from build123d import *

# Parameters (mm, degrees)
F0_W     = 77.2
F0_H     = 152.5
F1_DEPTH = 10.9
F2_R     = 10
F3_R     = 8
F4_R     = 1


with BuildPart() as f1:
    # F0 (on Top) → F1 (new body)
    with BuildSketch(Plane.XY):
        Rectangle(F0_W, F0_H)
    extrude(amount=F1_DEPTH)

    # F2
    f2_edges = [f1.edges().sort_by_distance(p)[0] for p in [
        (38.6, 76.25, 5.45),
        (-38.6, 76.25, 5.45),
        (-38.6, -76.25, 5.45),
        (38.6, -76.25, 5.45),
    ]]
    fillet(f2_edges, radius=F2_R)

    # F3
    f3_edges = [f1.edges().sort_by_distance(p)[0] for p in [
        (0, -76.25, 10.9),
        (-35.671068, -73.321068, 10.9),
        (35.671068, -73.321068, 10.9),
        (-38.6, 0, 10.9),
        (38.6, 0, 10.9),
        (-35.671068, 73.321068, 10.9),
        (35.671068, 73.321068, 10.9),
        (0, 76.25, 10.9),
    ]]
    fillet(f3_edges, radius=F3_R)

    # F4
    f4_edges = [f1.edges().sort_by_distance(p)[0] for p in [
        (0, -76.25, 0),
        (-35.671068, -73.321068, 0),
        (35.671068, -73.321068, 0),
        (-38.6, 0, 0),
        (38.6, 0, 0),
        (-35.671068, 73.321068, 0),
        (35.671068, 73.321068, 0),
        (0, 76.25, 0),
    ]]
    fillet(f4_edges, radius=F4_R)


solid = f1.part
Geometry: final body of the model. Coordinates: model frame, mm. Coordinates: 2 decimals unless noted, no trailing zeros. Loops run counter-clockwise (first coordinate to the right, second up) from the corner with the lowest first, then second, coordinate; pieces in that order, holes last. Notation, with made-up numbers: (13, 80.5) - (28, 80.5) arc R8 cw to (28, 89.5) - close; hole circle Ø11 at (-18, -18.5). An arc over 180 degrees is marked (long way). Put each result on its own line as item: value. Start each with the question number.
Q1. Cut plane B-B, the plane y = -16. Return loops of the section in (x, z).
Q2. Cut plane A-A, the plane x = 27. Return loops of the section in (y, z), and give its area (3 significant figures).
Q3. Line query: line 1 (X direction, y = -59, z = 3.25); line 2 (Z direction, x = -31, y = 49); line 3 (X direction, y = -36.5, z = 7.25). Output: solid intervals per line, ascending.
Filled sheet:
1. outline: (-38.6, 1) arc R1 ccw to (-37.6, 0) - (37.6, 0) arc R1 ccw to (38.6, 1) - (38.6, 2.9) arc R8 ccw to (30.6, 10.9) - (-30.6, 10.9) arc R8 ccw to (-38.6, 2.9) - close
2. outline: (-76.25, 1) arc R1 ccw to (-75.25, 0) - (75.25, 0) arc R1 ccw to (76.25, 1) - (76.25, 2.9) arc R8 ccw to (68.25, 10.9) - (-68.25, 10.9) arc R8 ccw to (-76.25, 2.9) - close
2. area: 1,630 mm²
3. line 1: -38.59 to 38.59
3. line 2: 0 to 10.89
3. line 3: -37.31 to 37.31
